The listing builds one solid part. Answer for the finished solid, in the listing's coordinates (mm). Round coordinates to 2 decimals unless told otherwise and drop trailing zeros. Order: outer loops, then holes, each group sorted by start corner. A loop starts at its lowest first (then second) coordinate and runs counter-clockwise, first axis right, second up. Notation, with made-up numbers: (-14.5, 27.25) - (7.5, 27.25) arc R32 cw to (7.5, 64.25) - close; hole circle Ø11 at (54, 31.5). An arc over 180 degrees is marked (long way). Write item = value, one per line.
Autodesk Inventor part; units mm, degrees
ref_plane "YZ Plane" through (0, 0, 0) normal (1, 0, 0) x (0, 1, 0)
ref_plane "XZ Plane" through (0, 0, 0) normal (0, 1, 0) x (-1, 0, 0)
ref_plane "XY Plane" through (0, 0, 0) normal (0, 0, 1) x (1, 0, 0)
sketch "Sketch1" plane through (0, 0, 0) normal (0, 0, 1) x (1, 0, 0)
  circle A0 centre (0, 0) radius 3.175
  circle A1 centre (0, 0) radius 2.675
  dimension "d0" = 6.35
  dimension "d1" = 5.35
extrude "Extrusion1" add sketch "Sketch1" along normal blind 342.525
sketch "Sketch2" plane through (0, 0, 342.525) normal (0, 0, 1) x (1, 0, 0)
  circle A0 centre (0, 0) radius 2.675
  circle A1 centre (0, 0) radius 3.175
extrude "Extrusion2" add sketch "Sketch2" along normal blind 30.87
sketch "Sketch3" plane through (0, 0, 373.395) normal (0, 0, 1) x (1, 0, 0)
  circle A0 centre (0, 0) radius 2.675
  circle A1 centre (0, 0) radius 3.175
extrude "Extrusion3" cut sketch "Sketch3" against normal blind 9.525
properties part number "coverplate pipe"
Q1. Section B-B on y = 1.5 is taken. Determine the outline of the cut face in (x, z).
Model answer:
outline = (-2.8, 0) - (-2.21, 0) - (-2.21, 363.87) - (-2.8, 363.87) - close; (2.21, 0) - (2.8, 0) - (2.8, 363.87) - (2.21, 363.87) - close
Q2. Section A-A on x = 0 is taken. Determine the outline of the cut face in (y, z) (3 decimals).
Model answer:
outline = (-3.175, 0) - (-2.675, 0) - (-2.675, 363.87) - (-3.175, 363.87) - close; (2.675, 0) - (3.175, 0) - (3.175, 363.87) - (2.675, 363.87) - close
Q3. Flat-ended cylindrical pins translate along their axes: P1, Ø3, axis at x = -0.5, z = 269.5, coming from the -Y side (3 decimals); P2, Ø1, axis at x = -1, z = 234, coming from the -Y side; P3, Ø3, axis at x = -2.5, z = 206, coming from the -Y side; P4, Ø1.5, axis at y = 1.5, z = 323.5, coming from the +X side. Find the tip coordinate at first contact, or state that the pin passes through.
Model answer:
P1 = -3.175
P2 = -3.14
P3 = -3.01
P4 = 3.09
Q4. Section C-C on z = 45.5 is taken. Determine the outline of the cut face in (x, y) (3 decimals), then the cut area to 3 significant figures.
Model answer:
outline = circle Ø6.35 at (0, 0); hole circle Ø5.35 at (0, 0)
area = 9.19 mm^2
Q5. Find the intervals of material crossed by line 1 (Y direction, x = 0, z = 133) (3 decimals); line 2 (Y direction, x = -0.5, z = 218); line 3 (X direction, y = 1.75, z = 295), in increasing order. Write a range as from..to.
Model answer:
line_1 = -3.175..-2.675, 2.675..3.175
line_2 = -3.14..-2.63, 2.63..3.14
line_3 = -2.65..-2.02, 2.02..2.65
